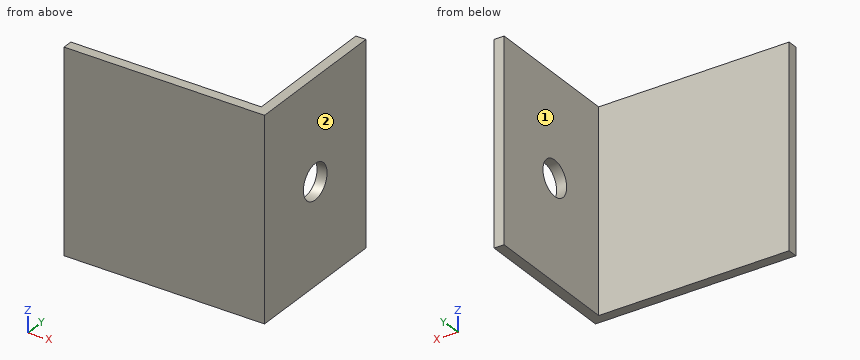
```python
from build123d import *

# Parameters (mm, degrees)
SALIENTE_EXTRUIR1_DEPTH = 40
CROQUIS2_R              = 3.5
CORTAR_EXTRUIR1_DEPTH   = 64.2003722


with BuildPart() as part:
    # Croquis1 → Saliente-Extruir1 (new body)
    with BuildSketch(Plane.XY):
        Polygon((0.551367026, 28.183098592), (0.551367026, -1.816901408), (-39.448632974, -1.816901408), (-39.448632974, 0.183098592), (-1.448632974, 0.183098592), (-1.448632974, 28.183098592), align=None)
    extrude(amount=SALIENTE_EXTRUIR1_DEPTH)

    # Croquis2 → Cortar-Extruir1 (cut, through all)
    with BuildSketch(Plane(origin=(0.551367026, 0, 0), x_dir=(0, 0, -1), z_dir=(1, 0, 0))):
        with Locations(Location((-20, 13.183098592, 0), (0, 0, 90))):
            Circle(CROQUIS2_R)
    extrude(amount=-CORTAR_EXTRUIR1_DEPTH, mode=Mode.SUBTRACT)


solid = part.part
```
The listing builds one solid part. Answer for the finished solid, in the listing's coordinates (mm). Face numbers are marked on the shaded views. A direction names the side the tool comes from. Give positions to 0.01 mm unless a question says otherwise; leave off trailing zeros. Order: outer loops, then holes, each group sorted by start corner. A loop starts at its lowest first (then second) coordinate and runs counter-clockwise, first axis right, second up.
1) Find section B-B on y = 15.25. Write down the section's boundary in (x, z), then the cut area to 3 significant figures.
Reported:
outline: (-1.45, 0) - (0.55, 0) - (0.55, 17.18) - (-1.45, 17.18) - close; (-1.45, 22.82) - (0.55, 22.82) - (0.55, 40) - (-1.45, 40) - close
area: 68.7 mm2
2) Find section D-D on x = -24. Write down the section's boundary in (y, z).
Reported:
outline: (-1.82, 0) - (0.18, 0) - (0.18, 40) - (-1.82, 40) - close
3) Find section A-A on z = 20. Write down the section's boundary in (x, y).
Reported:
outline: (-39.45, -1.82) - (0.55, -1.82) - (0.55, 9.68) - (-1.45, 9.68) - (-1.45, 0.18) - (-39.45, 0.18) - close; (-1.45, 16.68) - (0.55, 16.68) - (0.55, 28.18) - (-1.45, 28.18) - close
4) Consider line 1 along X through (y, z) = (25.25, 28); line 2 along Y through (x, z) = (-6.5, 2). Determine where each line is inside the solid, lowest interval first.
Reported:
line 1: x = -1.45 to 0.55
line 2: y = -1.82 to 0.18
5) Find section C-C on z = 36.5. Write down the section's boundary in (x, y), then the cut area to 3 significant figures.
Reported:
outline: (-39.45, -1.82) - (0.55, -1.82) - (0.55, 28.18) - (-1.45, 28.18) - (-1.45, 0.18) - (-39.45, 0.18) - close
area: 136 mm2
6) For the marked faces 1 and 2, determine the directions among +Z, -Z, +X, -X, +Y, -Y from which every point of the face is accessible in a straight line to the end or side of a thin tool.
Reported:
face 1: +Z, -Z, -X, +Y
face 2: +Z, -Z, +X, +Y, -Y
7) Given P1, Ø1, axis at x = -31, z = 15, coming from the +Y side; P2, Ø11, axis at y = 13.18, z = 20, coming from the -X side, each flat-ended and moving along its own axis, determine where each tip first touches the part or whether it passes through.
Reported:
P1: stops at y = 0.18
P2: stops at x = -1.45
